The listing builds one solid part. Answer for the finished solid, in the listing's coordinates (mm). Coordinates: 2 decimals unless noted, no trailing zeros. Write each loop counter-clockwise with the first axis right and the second up, starting at its lowest first coordinate (ties: lowest second). Pieces come first, ordered by that corner, then holes.
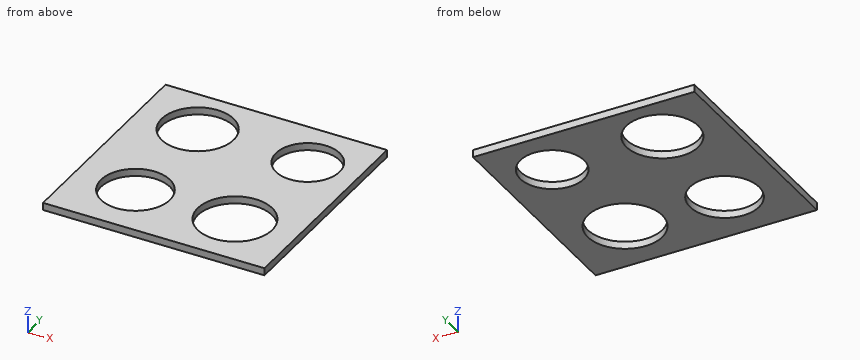
from build123d import *

# Parameters (mm, degrees)
SKETCH1_W           = 30
SKETCH1_H           = 30
BOSS_EXTRUDE1_DEPTH = 1
SKETCH2_R           = 4.316163829
CUT_EXTRUDE1_DEPTH  = 3
SKETCH3_R           = 5.043132961
CUT_EXTRUDE2_DEPTH  = 3
SKETCH4_R           = 4.877423457
CUT_EXTRUDE3_DEPTH  = 3
SKETCH5_R           = 4.666431363
CUT_EXTRUDE4_DEPTH  = 3


with BuildPart() as part:
    # Sketch1 → Boss-Extrude1 (new body)
    with BuildSketch(Plane.XY):
        Rectangle(SKETCH1_W, SKETCH1_H)
    extrude(amount=BOSS_EXTRUDE1_DEPTH)

    # Sketch2 → Cut-Extrude1 (cut)
    with BuildSketch(Plane(origin=(0, 0, 0), x_dir=(-1, 0, 0), z_dir=(0, 0, -1))):
        with Locations((-8.12429837, 8.038997658)):
            Circle(SKETCH2_R)
    extrude(amount=-CUT_EXTRUDE1_DEPTH, mode=Mode.SUBTRACT)

    # Sketch3 → Cut-Extrude2 (cut)
    with BuildSketch(Plane(origin=(0, 0, 0), x_dir=(-1, 0, 0), z_dir=(0, 0, -1))):
        with Locations((-6.650270789, -7.131419922)):
            Circle(SKETCH3_R)
    extrude(amount=-CUT_EXTRUDE2_DEPTH, mode=Mode.SUBTRACT)

    # Sketch4 → Cut-Extrude3 (cut)
    with BuildSketch(Plane(origin=(0, 0, 0), x_dir=(-1, 0, 0), z_dir=(0, 0, -1))):
        with Locations((6.8674749, 8.16200162)):
            Circle(SKETCH4_R)
    extrude(amount=-CUT_EXTRUDE3_DEPTH, mode=Mode.SUBTRACT)

    # Sketch5 → Cut-Extrude4 (cut)
    with BuildSketch(Plane(origin=(0, 0, 0), x_dir=(-1, 0, 0), z_dir=(0, 0, -1))):
        with Locations((6.808728507, -7.165302377)):
            Circle(SKETCH5_R)
    extrude(amount=-CUT_EXTRUDE4_DEPTH, mode=Mode.SUBTRACT)


solid = part.part
1. Section B-B on x = -8.5 is taken. Give the vertices of the cut face in (y, z).
Results found:
outline: (-15, 0) - (-11.51, 0) - (-11.51, 1) - (-15, 1) - close; (-2.82, 0) - (3.57, 0) - (3.57, 1) - (-2.82, 1) - close; (12.76, 0) - (15, 0) - (15, 1) - (12.76, 1) - close
2. Find the intervals of material crossed by L1, parallel to Y at x = 11, z = 0.25; L2, parallel to X at y = -4, z = 0.1; L3, parallel to X at y = -4.5, z = 0.35, in increasing order.
Results found:
L1: y = -15 to -9.68, -4.58 to 4.82, 11.26 to 15
L2: x = -15 to -10.24, -3.38 to 2.7, 10.6 to 15
L3: x = -15 to -10.64, -2.98 to 2.35, 10.95 to 15
3. Section C-C on z = 0.35 is taken. Give the vertices of the cut face in (x, y), then the cut area to 3 significant figures.
Results found:
outline: (-15, -15) - (15, -15) - (15, 15) - (-15, 15) - close; hole circle Ø9.75 at (-6.87, 8.16); hole circle Ø9.33 at (-6.81, -7.17); hole circle Ø10.09 at (6.65, -7.13); hole circle Ø8.63 at (8.12, 8.04)
area: 618 mm2
4. Section A-A on y = 8.75 is taken. Give the vertices of the cut face in (x, z).
Results found:
outline: (-15, 0) - (-11.71, 0) - (-11.71, 1) - (-15, 1) - close; (-2.03, 0) - (3.87, 0) - (3.87, 1) - (-2.03, 1) - close; (12.38, 0) - (15, 0) - (15, 1) - (12.38, 1) - close
5. A flat-ended cylindrical pin translates along its axis: P1, Ø7, axis at x = 8.12, y = 8.04, coming from the +Z side. Find the tip coordinate at first contact, or state that the pin passes through.
Results found:
P1: passes through
